from build123d import *

# Parameters (mm, degrees)
CHAMFER_2_SIZE      = 2
FILLET_2_R          = 0.6
SKETCH_7_OUTSIDE_W  = 32.128
SKETCH_7_OUTSIDE_H  = 32.128
CUT_EXTRUDE_5_DEPTH = 7


with BuildPart() as part:
    # Эскиз1 → Повернуть2 (revolve)
    with BuildSketch(Plane(origin=(0, 0, 0), x_dir=(0, 0, -1), z_dir=(1, 0, 0)), mode=Mode.PRIVATE) as revolve_2_sk:
        Polygon((0, 8), (0, 0), (42, 0), (42, 6), (7, 6), (7, 10), (1.154700538, 10), align=None)
    revolve(revolve_2_sk.sketch.rotate(Axis((0, 0, 0), (0, 0, -1)), 90), axis=Axis((0, 0, 0), (0, 0, -1)))

    # Фаска2
    chamfer_2_edges = [part.edges().sort_by_distance(p)[0] for p in [
        (-6, 0, -42),
    ]]
    chamfer(chamfer_2_edges, length=CHAMFER_2_SIZE)

    # Скругление2
    fillet_2_edges = [part.edges().sort_by_distance(p)[0] for p in [
        (-6, 0, -7),
    ]]
    fillet(fillet_2_edges, radius=FILLET_2_R)

    # Эскиз7 outside → Вырез-Вытянуть5 (cut)
    with BuildSketch(Plane.XY):
        Rectangle(SKETCH_7_OUTSIDE_W, SKETCH_7_OUTSIDE_H)
        Polygon((0, 9.814954576), (-8.5, 4.907477288), (-8.5, -4.907477288), (0, -9.814954576), (8.5, -4.907477288), (8.5, 4.907477288), align=None, mode=Mode.SUBTRACT)
    extrude(amount=-CUT_EXTRUDE_5_DEPTH, mode=Mode.SUBTRACT)


solid = part.part
Model file for the job. Use its own axes, mm. Give positions to 0.01 mm unless a question says otherwise; leave off trailing zeros. Write each loop counter-clockwise with the first axis right and the second up, starting at its lowest first coordinate (ties: lowest second). Pieces come first, ordered by that corner, then holes. Notation, with made-up numbers: M 23.5,47 L 50.5,47 A18 ccw 50.5,79 Z; hole C 43,32.5 d6. An arc over 180 degrees is marked long. One line per item, written item: value. Start each with the question number.
Q1. Saw through at A-A, the plane y = 0. Write the cut outline in (x, z), plus the area to 3 significant figures.
Q2. Drop flat-ended pins along their axis: pin 1 Ø6 at (y, z) = (-4, -31.5) entering from -X; pin 2 Ø10 at (x, z) = (-2.5, -16) entering from +Y; pin 3 Ø5 at (y, z) = (7, -31.5) entering from -X. Give the stop position or say it passes through.
Q3. Two-plate mould, pull along Y, no slides. Class faces 1 (the flat face through (-1.85, 6.5, -7)), 2 (the flat face through (4.309, 7.327, -3.597)), 3 (the cylindrical face through (5.723, -1.802, -23.573)): +Y half, -Y half, draft (parallel to the pull), parting line (faces both ways), or undercut.
Q4. Saw through at B-B, the plane z = -26. Write the cut outline in (x, y), plus the area to 3 significant figures.
Q5. Probe probe 1 along Z at (x, y) = (0.25, 7.75); probe 2 along X at (y, z) = (5, -1.5); probe 3 along X at (y, z) = (6.5, -5). List the from-to ranges inside material, lowest first. Write a range as [from, to].
Output values:
1. outline: M -8.5,-7 L -6.6,-7 A0.6 cw -6,-7.6 L -6,-40 L -4,-42 L 4,-42 L 6,-40 L 6,-7.6 A0.6 cw 6.6,-7 L 8.5,-7 L 8.5,-0.29 L 8,0 L -8,0 L -8.5,-0.29 Z
1. area: 535 mm²
2. pin 1: stops at x = -5.92
2. pin 2: stops at y = 6
2. pin 3: stops at x = -3.97
3. face 1: draft
3. face 2: +Y half
3. face 3: parting line
4. outline: C 0,0 d12
4. area: 113 mm²
5. probe 1: z = [-7, 0]
5. probe 2: x = [-8.34, 8.34]
5. probe 3: x = [-5.74, 5.74]
